Verification items for the finished model (mm, model axes). A direction names the side the tool comes from. Coordinates: 2 decimals unless noted, no trailing zeros. Loops run counter-clockwise (first coordinate to the right, second up) from the corner with the lowest first, then second, coordinate; pieces in that order, holes last. Notation, with made-up numbers: (74.25, 17) - (97.25, 17) arc R31 ccw to (97.25, 45) - close; hole circle Ø2 at (64, 50.5). An arc over 180 degrees is marked (long way). Answer as CSV lines item,"result". Start each with the question number.
1. Material ranges on line 1 (X direction, y = 6, z = 13); line 2 (Y direction, x = 95.75, z = 29.15); line 3 (Z direction, x = 92, y = 19), recorded low to high. Write a range as [from, to].
2. Cross-section at A-A (x = 69.35). Enter the section's corners in (y, z), plus the area to 3 significant figures.
3. Release check for a two-part mould opening along Z. For faces 3 (the flat face through (0, 6, 21)), 4 (the flat face through (65, 11, 0)), 5 (the flat face through (65, 11, 42.3)), 6 (the cylindrical face through (24.07, 5.73, 28.53)) record: pulls with the +Z half, pulls with the -Z half, needs draft (parallel to the pull), parting line crosses it, or undercut.
4. Cross-section at D-D (z = 20). Enter the section's corners in (x, y), plus the area to 3 significant figures.
5. Cross-section at B-B (z = 13.15). Enter the section's corners in (x, y).
6. Set-up check for faces 1 (the cylindrical face through (64.7, 5.73, 28.12)), 2 (the flat face through (88.7, 38, 21)): record each of +Z, -Z, +X, -X, +Y, -Y from which the full face is reachable in a straight line by a thin tool's end or side.
7. Cross-section at C-C (y = 52.5). Enter the section's corners in (x, z).
8. Gauge pin test, flat ends, axial feed: P1, Ø4, axis at x = 58.5, z = 33.5, coming from the +Y side; P2, Ø8, axis at y = 42.5, z = 7, coming from the -X side. Record the tip position at first contact, or that the pin passes through.
```python
from build123d import *

# Parameters (mm, degrees)
SKETCH1_W           = 100
SKETCH1_H           = 42.3
BOSS_EXTRUDE1_DEPTH = 11.3
SKETCH2_W           = 11.3
SKETCH2_H           = 42.3
BOSS_EXTRUDE2_DEPTH = 53.7
SKETCH3_R           = 4.7625
CUT_EXTRUDE1_DEPTH  = 53.7
SKETCH4_R           = 4.7625
CUT_EXTRUDE2_DEPTH  = 53.7


with BuildPart() as part:
    # Sketch1 → Boss-Extrude1 (new body)
    with BuildSketch(Plane(origin=(0, 0, 0), x_dir=(1, 0, 0), z_dir=(0, 1, 0))):
        with Locations((50, -21.15)):
            Rectangle(SKETCH1_W, SKETCH1_H)
    extrude(amount=BOSS_EXTRUDE1_DEPTH)

    # Sketch2 → Boss-Extrude2 (add)
    with BuildSketch(Plane(origin=(0, 11.3, 0), x_dir=(1, 0, 0), z_dir=(0, 1, 0))):
        with Locations((94.35, -21.15)):
            Rectangle(SKETCH2_W, SKETCH2_H)
    extrude(amount=BOSS_EXTRUDE2_DEPTH)

    # Sketch3 → Cut-Extrude1 (cut)
    with BuildSketch(Plane(origin=(100, 0, 0), x_dir=(0, 0, -1), z_dir=(1, 0, 0))):
        with Locations((-13.15, 22.5)):
            Circle(SKETCH3_R)
        with Locations((-13.15, 52.5)):
            Circle(SKETCH3_R)
        with Locations((-29.15, 52.5)):
            Circle(SKETCH3_R)
        with Locations((-29.15, 22.5)):
            Circle(SKETCH3_R)
    extrude(amount=-CUT_EXTRUDE1_DEPTH, mode=Mode.SUBTRACT)

    # Sketch4 → Cut-Extrude2 (cut)
    with BuildSketch(Plane(origin=(0, 11.3, 0), x_dir=(1, 0, 0), z_dir=(0, 1, 0))):
        with Locations(Location((19.35, -13.15, 0), (0, 0, 270))):
            Circle(SKETCH4_R)
        with Locations(Location((69.35, -13.15, 0), (0, 0, 270))):
            Circle(SKETCH4_R)
        with Locations(Location((19.35, -29.15, 0), (0, 0, 270))):
            Circle(SKETCH4_R)
        with Locations(Location((69.35, -29.15, 0), (0, 0, 270))):
            Circle(SKETCH4_R)
    extrude(amount=-CUT_EXTRUDE2_DEPTH, mode=Mode.SUBTRACT)


solid = part.part
```
Values follow:
1,line 1,"x = [0, 14.59], [24.11, 64.59], [74.11, 100]"
1,line 2,"y = [0, 17.74], [27.26, 47.74], [57.26, 65]"
1,line 3,"z = [0, 9.92], [16.38, 25.92], [32.38, 42.3]"
2,outline,"(0, 0) - (11.3, 0) - (11.3, 8.39) - (0, 8.39) - close; (0, 17.91) - (11.3, 17.91) - (11.3, 24.39) - (0, 24.39) - close; (0, 33.91) - (11.3, 33.91) - (11.3, 42.3) - (0, 42.3) - close"
2,area,"263 mm²"
3,face 3,"needs draft"
3,face 4,"pulls with the -Z half"
3,face 5,"pulls with the +Z half"
3,face 6,"undercut"
4,outline,"(0, 0) - (100, 0) - (100, 65) - (88.7, 65) - (88.7, 11.3) - (0, 11.3) - close"
4,area,"1,740 mm²"
5,outline,"(0, 0) - (14.59, 0) - (14.59, 11.3) - (0, 11.3) - close; (24.11, 0) - (64.59, 0) - (64.59, 11.3) - (24.11, 11.3) - close; (74.11, 0) - (100, 0) - (100, 17.74) - (88.7, 17.74) - (88.7, 11.3) - (74.11, 11.3) - close; (88.7, 27.26) - (100, 27.26) - (100, 47.74) - (88.7, 47.74) - close; (88.7, 57.26) - (100, 57.26) - (100, 65) - (88.7, 65) - close"
6,face 1,"+Y, -Y"
6,face 2,"+Z, -Z, -X, +Y"
7,outline,"(88.7, 0) - (100, 0) - (100, 8.39) - (88.7, 8.39) - close; (88.7, 17.91) - (100, 17.91) - (100, 24.39) - (88.7, 24.39) - close; (88.7, 33.91) - (100, 33.91) - (100, 42.3) - (88.7, 42.3) - close"
8,P1,"stops at y = 11.3"
8,P2,"stops at x = 88.7"
